Read the model definition and answer for the solid it produces. Units are mm, in the model's axes. Face numbers are marked on the shaded views. Coordinates: 2 decimals unless noted, no trailing zeros. Loops run counter-clockwise (first coordinate to the right, second up) from the corner with the lowest first, then second, coordinate; pieces in that order, holes last.
Autodesk Inventor part; units mm, degrees
ref_plane "YZ Plane" through (0, 0, 0) normal (1, 0, 0) x (0, 1, 0)
ref_plane "XZ Plane" through (0, 0, 0) normal (0, 1, 0) x (-1, 0, 0)
ref_plane "XY Plane" through (0, 0, 0) normal (0, 0, 1) x (1, 0, 0)
sketch "Sketch1" plane through (0, 0, 0) normal (0, 1, 0) x (-1, 0, 0)
  circle A0 centre (0, 0) radius 4.1
  circle A1 centre (0, 0) radius 11
  dimension "d0" = 8.2
  dimension "d1" = 22
extrude "Extrusion1" add sketch "Sketch1" along normal blind 4
sketch "Sketch2" plane through (0, 4, 0) normal (0, 1, 0) x (1, 0, 0)
  line L0 (0, 0) -> (-8.1688, -0.7147) construction
  line L1 (0, 0) -> (-8.1688, 0.7147) construction
  arc A0 (-4.0844, 0.3573) -> (-4.0844, -0.3573) centre (10.5368, 0) ccw
  line L2 (-4.0844, 0.3573) -> (-10.9581, 0.9587)
  line L3 (-15.4, 0) -> (15.4, 0) construction
  circle A1 centre (0, 0) radius 4.1 construction
  circle A2 centre (0, 0) radius 11 construction
  line L4 (-4.0844, -0.3573) -> (-10.9581, -0.9587)
  circle A3 centre (0, 0) radius 11
  dimension "d4" = 10
extrude "Extrusion2" add sketch "Sketch2" along normal blind 2 contours A0 L4 A3 L2 picked at (-8.693, 0.0397)
sketch "Sketch3" plane through (0, 0, 0) normal (0, 0, 1) x (1, 0, 0)
  circle A0 centre (0, 2) radius 1.25
  line L0 (11, 0) -> (-11, 0)
  point P0 (0, 0)
  dimension "d7" = 2.5
  dimension "d8" = 2
extrude "Extrusion3" cut sketch "Sketch3" against normal through all both and the other way through all
properties part number "10d_coupler"
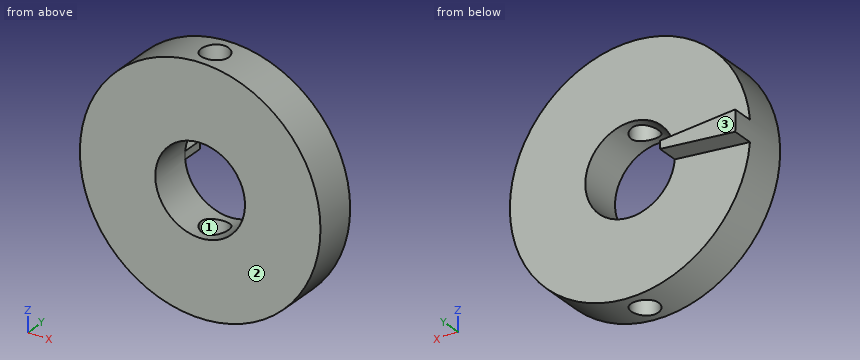
Q1. A cutting plane is placed at D-D (z = 5.5). Give the vertices of the cut face in (x, y), then the cut area to 3 significant figures.
Findings below:
outline: (-9.53, 0) - (9.53, 0) - (9.53, 4) - (-9.53, 4) - close; hole circle Ø2.5 at (0, 2)
area: 71.3 mm2
Q2. A cutting plane is placed at A-A (x = 0). Give the vertices of the cut face in (y, z), then the cut area to 3 significant figures.
Findings below:
outline: (0, -11) - (0.75, -11) - (0.75, -4.1) - (0, -4.1) - close; (0, 4.1) - (0.75, 4.1) - (0.75, 11) - (0, 11) - close; (3.25, -11) - (4, -11) - (4, -4.1) - (3.25, -4.1) - close; (3.25, 4.1) - (4, 4.1) - (4, 11) - (3.25, 11) - close
area: 20.7 mm2
Q3. Flat-ended cylindrical pins translate along their axes: pin 1 Ø6.5 at (x, z) = (0, 0) entering from +Y; pin 2 Ø2 at (x, z) = (-2, -7) entering from +Y; pin 3 Ø1.5 at (x, y) = (-5, 4.5) entering from -Z; pin 4 Ø11 at (x, z) = (-2, 4.5) entering from +Y. Find the tip coordinate at first contact, or state that the pin passes through.
Findings below:
pin 1: passes through
pin 2: stops at y = 4
pin 3: stops at z = -10.06
pin 4: stops at y = 6
Q4. A cutting plane is placed at B-B (y = 2). Give the vertices of the cut face in (x, z), then the cut area to 3 significant figures.
Findings below:
outline: (-1.25, -10.93) - (-1.25, -3.9) arc R4.1 cw to (-1.25, 3.9) - (-1.25, 10.93) arc R11 ccw to start; (1.25, -10.93) arc R11 ccw to (1.25, 10.93) - (1.25, 3.9) arc R4.1 cw to (1.25, -3.9) - close
area: 293 mm2
Q5. Determine the mould class of the marked faces 1, 2 and 3 for opening direction Y: +Y half, -Y half, draft (parallel to the pull), parting line (faces both ways), or undercut.
Findings below:
face 1: undercut
face 2: -Y half
face 3: +Y half
Q6. Straight lines are drawn through the part: probe 1 along Y at (x, z) = (0, 9.5); probe 2 along X at (y, z) = (1, -7.75); probe 3 along Z at (x, y) = (-2, 3.5). For each, find the intervals that lie inside material, in ascending order.
Findings below:
probe 1: y = 0 to 0.75, 3.25 to 4
probe 2: x = -7.81 to -0.75, 0.75 to 7.81
probe 3: z = -10.82 to -3.58, 3.58 to 10.82
Q7. A cutting plane is placed at C-C (x = -3.25). Give the vertices of the cut face in (y, z).
Findings below:
outline: (0, -10.51) - (4, -10.51) - (4, -2.5) - (0, -2.5) - close; (0, 2.5) - (4, 2.5) - (4, 10.51) - (0, 10.51) - close
